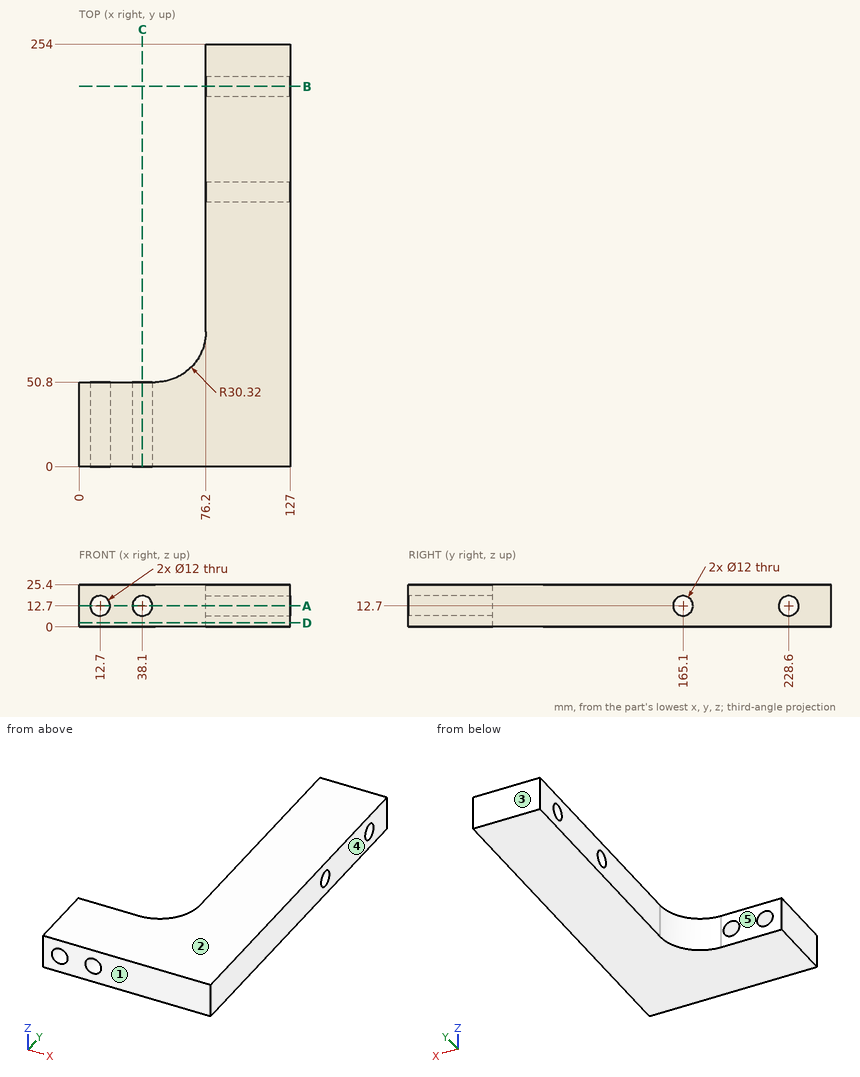
The figure shows three views and two pictorial views of one solid part (mm, origin at its lowest corner). Answer the questions. A direction names the side the tool comes from. Coordinates: 2 decimals unless noted, no trailing zeros. Loops run counter-clockwise (first coordinate to the right, second up) from the corner with the lowest first, then second, coordinate; pieces in that order, holes last. Notation, with made-up numbers: (22, 25) - (74, 25) arc R23 cw to (74, 44) - close; hole circle Ø3 at (68.25, 15). An arc over 180 degrees is marked (long way). Use a Markdown table: item, result. Add a question column.
1) The part is cut by section B-B, the plane y = 228.6. Give the vertices of the cut face in (x, z), and give its area (3 significant figures).
2) Given pin 1 (5 mm diameter, centred on x = 41.5, z = 9.5, fed in from +Y); pin 2 (11 mm diameter, centred on y = 165.1, z = 12.7, fed in from -X); pin 3 (10 mm diameter, centred on x = 109, y = 111, fed in from -Z); pin 4 (4 mm diameter, centred on y = 139.5, z = 5.5, fed in from -X), each flat-ended and moving along its own axis, determine where each tip first touches the part or whether it passes through.
3) The part is cut by section D-D, the plane z = 2.5. Give the vertices of the cut face in (x, y), and give its area (3 significant figures).
4) The mould has two halves that part along Y. Classify the marked faces 1, 2 and 3: released by +Y, released by -Y, zero draft, split by the parting line, or undercut.
5) The part is cut by section A-A, the plane z = 12.7. Give the vertices of the cut face in (x, y).
6) Find the intervals of material crossed by line 1 (Y direction, x = 105, z = 12.7); line 2 (Z direction, x = 102, y = 228); line 3 (Y direction, x = 110.5, z = 11), in increasing order.
7) For the marked faces 4 and 5, determine the directions among +Z, -Z, +X, -X, +Y, -Y from which every point of the face is accessible in a straight line to the end or side of a thin tool.
8) The part is cut by section C-C, the plane x = 38.1. Give the vertices of the cut face in (y, z), and give its area (3 significant figures).
Here are the results:
| question | item | result |
|---|---|---|
| 1 | outline | (76.2, 0) - (127, 0) - (127, 6.7) - (76.2, 6.7) - close; (76.2, 18.7) - (127, 18.7) - (127, 25.4) - (76.2, 25.4) - close |
| 1 | area | 681 mm^2 |
| 2 | pin 1 | stops at y = 50.8 |
| 2 | pin 2 | passes through |
| 2 | pin 3 | stops at z = 0 |
| 2 | pin 4 | stops at x = 76.2 |
| 3 | outline | (0, 0) - (127, 0) - (127, 254) - (76.2, 254) - (76.2, 81.12) arc R30.32 cw to (45.88, 50.8) - (0, 50.8) - close |
| 3 | area | 17,000 mm^2 |
| 4 | face 1 | released by -Y |
| 4 | face 2 | zero draft |
| 4 | face 3 | released by +Y |
| 5 | outline | (0, 0) - (6.7, 0) - (6.7, 50.8) - (0, 50.8) - close; (18.7, 0) - (32.1, 0) - (32.1, 50.8) - (18.7, 50.8) - close; (44.1, 0) - (127, 0) - (127, 159.1) - (76.2, 159.1) - (76.2, 81.12) arc R30.32 cw to (45.88, 50.8) - (44.1, 50.8) - close; (76.2, 171.1) - (127, 171.1) - (127, 222.6) - (76.2, 222.6) - close; (76.2, 234.6) - (127, 234.6) - (127, 254) - (76.2, 254) - close |
| 6 | line 1 | y = 0 to 159.1, 171.1 to 222.6, 234.6 to 254 |
| 6 | line 2 | z = 0 to 6.73, 18.67 to 25.4 |
| 6 | line 3 | y = 0 to 159.35, 170.85 to 222.85, 234.35 to 254 |
| 7 | face 4 | +Z, -Z, +X, +Y, -Y |
| 7 | face 5 | +Z, -Z, -X, +Y |
| 8 | outline | (0, 0) - (50.8, 0) - (50.8, 6.7) - (0, 6.7) - close; (0, 18.7) - (50.8, 18.7) - (50.8, 25.4) - (0, 25.4) - close |
| 8 | area | 681 mm^2 |
